CAD build for the part. Positions are in the model's coordinates, mm. Face numbers are marked on the shaded views. A direction names the side the tool comes from. Give positions to 0.01 mm unless a question says otherwise; leave off trailing zeros. Loops run counter-clockwise (first coordinate to the right, second up) from the corner with the lowest first, then second, coordinate; pieces in that order, holes last.
Item 1: Mould opens along Z. For the marked faces 1, 2 and 3 say: released by +Z, released by -Z, zero draft, split by the parting line, or undercut.
Item 2: Which spindle directions (+Z, -Z, +X, -X, +Y, -Y) get a long thin tool onto all of the face, cutting with end or side? Do the marked faces 4 and 5. Say none if no direction does.
Item 3: Drop flat-ended pins along their axis: P1, Ø3, axis at x = 21, z = -6.5, coming from the +Y side; P2, Ø25, axis at y = 149, z = 11.5, coming from the +X side. Give the stop position or say it passes through.
Item 4: Saw through at D-D on z = -13. Give the cut face in (x, y), plus the area to 3 significant figures.
Item 5: Saw through at A-A on z = 0. Give the cut face in (x, y), plus the area to 3 significant figures.
Item 6: Probe probe 1 along Y at (x, z) = (3.5, 0); probe 2 along Y at (x, z) = (24, -13.5). List the from-to ranges inside material, lowest first.
Item 7: Saw through at C-C on x = 5.5. Give the cut face in (y, z).
Item 8: Saw through at B-B on y = 80. Give the cut face in (x, z), plus the area to 3 significant figures.
from build123d import *

# Parameters (mm, degrees)
BOSS_EXTRUDE1_DEPTH = 25
SKETCH2_R           = 4
CUT_EXTRUDE1_DEPTH  = 201.81085628
SKETCH3_R           = 4
CUT_EXTRUDE2_DEPTH  = 208.665596573
BOSS_EXTRUDE2_DEPTH = 10


with BuildPart() as part:
    # Sketch1 → Boss-Extrude1 (new, symmetric)
    with BuildSketch(Plane.XY):
        Polygon((0, 0), (0, 200), (10, 200), (10, 10), (60, 10), (60, 0), align=None)
    extrude(amount=BOSS_EXTRUDE1_DEPTH, both=True)

    # Sketch2 → Cut-Extrude1 (cut, through all)
    with BuildSketch(Plane(origin=(0, 10, 0), x_dir=(1, 0, 0), z_dir=(0, 1, 0))):
        with Locations(Location((30, 0, 0), (0, 0, 180))):
            Circle(SKETCH2_R)
    extrude(amount=-CUT_EXTRUDE1_DEPTH, mode=Mode.SUBTRACT)

    # Sketch3 → Cut-Extrude2 (cut, through all)
    with BuildSketch(Plane(origin=(10, 0, 0), x_dir=(0, 0, -1), z_dir=(1, 0, 0))):
        with Locations((0, 180)):
            Circle(SKETCH3_R)
        with Locations((0, 130)):
            Circle(SKETCH3_R)
        with Locations((0, 80)):
            Circle(SKETCH3_R)
    extrude(amount=-CUT_EXTRUDE2_DEPTH, mode=Mode.SUBTRACT)

    # Sketch5 → Boss-Extrude2 (add)
    with BuildSketch(Plane.XY.offset(25)):
        Polygon((10, 10), (30, 10), (10, 40), align=None)
    boss_extrude2 = extrude(amount=-BOSS_EXTRUDE2_DEPTH)

    # Mirror1: Boss-Extrude2 across plane
    add(boss_extrude2.mirror(Plane(origin=(0, 0, 0), x_dir=(1, 0, 0), z_dir=(0, 0, -1))))


solid = part.part
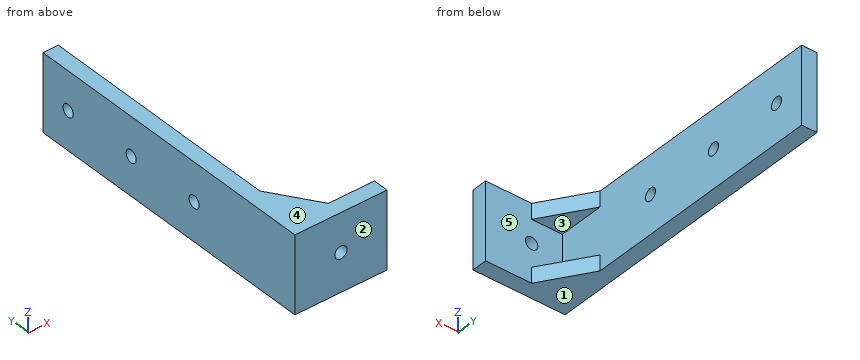
Results below:
1. face 1: released by -Z
1. face 2: zero draft
1. face 3: undercut
2. face 4: +Z, +X, -X, +Y, -Y
2. face 5: +X, +Y
3. P1: stops at y = 10
3. P2: stops at x = 10
4. outline: (0, 0) - (60, 0) - (60, 10) - (10, 10) - (10, 200) - (0, 200) - close
4. area: 2,500 mm2
5. outline: (0, 0) - (26, 0) - (26, 10) - (10, 10) - (10, 76) - (0, 76) - close; (0, 84) - (10, 84) - (10, 126) - (0, 126) - close; (0, 134) - (10, 134) - (10, 176) - (0, 176) - close; (0, 184) - (10, 184) - (10, 200) - (0, 200) - close; (34, 0) - (60, 0) - (60, 10) - (34, 10) - close
5. area: 2,180 mm2
6. probe 1: y = 0 to 76, 84 to 126, 134 to 176, 184 to 200
6. probe 2: y = 0 to 10
7. outline: (0, -25) - (200, -25) - (200, 25) - (0, 25) - close; hole circle Ø8 at (80, 0); hole circle Ø8 at (130, 0); hole circle Ø8 at (180, 0)
8. outline: (0, -25) - (10, -25) - (10, -4) - (0, -4) - close; (0, 4) - (10, 4) - (10, 25) - (0, 25) - close
8. area: 420 mm2
